Part model, mm, in its own coordinate system. A direction names the side the tool comes from. Round coordinates to 2 decimals unless told otherwise and drop trailing zeros. Write each loop counter-clockwise with the first axis right and the second up, starting at its lowest first coordinate (ties: lowest second). Pieces come first, ordered by that corner, then holes. Notation, with made-up numbers: (23, 71.5) -> (50, 71.5) arc R15 ccw to (50, 87.5) -> close; hole circle Ø10 at (-2.5, -38). An arc over 180 degrees is marked (long way). Use CSV: the item, a comma, the result in double quotes. Start each with the question number.
(1) Saw through at A-A (y = 231.5). Give the cut face in (x, z).
(2) Which spindle directions (+Z, -Z, +X, -X, +Y, -Y) get a long thin tool onto all of the face, cutting with end or side? Do faces 5 (the flat face through (51, 247, 0)), 6 (the flat face through (41.5, 321, 14)), 7 (the cylindrical face through (16.28, 46.49, 13.8)), 8 (the flat face through (61.5, 321, 14)). Say none if no direction does.
(3) Two-plate mould, pull along X, no slides. Class faces 1 (the flat face through (0, 24, 14)), 2 (the flat face through (51, 247, 28)), 3 (the flat face through (103, 24, 14)), 4 (the flat face through (51, 51, 14)): released by +X, released by -X, zero draft, split by the parting line, or undercut.
(4) Drop flat-ended pins along their axis: pin 1 (1.5 mm diameter, centred on x = 15.5, z = 17.5, fed in from -Y); pin 2 (14 mm diameter, centred on x = 59.5, z = 18.5, fed in from -Y); pin 3 (4 mm diameter, centred on x = 34.5, z = 3.5, fed in from +Y); pin 4 (5 mm diameter, centred on y = 8.5, z = 14, fed in from -X). Give the stop position or say it passes through.
(5) Probe line 1 (Z direction, x = 100, y = 8); line 2 (Y direction, x = 29, z = 20); line 3 (Y direction, x = 45.75, z = 14). List the from-to ranges inside material, lowest first. Write a range as [from, to].
```python
from build123d import *

# Parameters (mm, degrees)
BOSS_EXTRU_1_DEPTH      = 28
ESQUISSE2_R             = 3
ENL_V_MAT_EXTRU_1_DEPTH = 124.943535531
ESQUISSE3_W             = 20
ESQUISSE3_H             = 28
BOSS_EXTRU_2_DEPTH      = 524
CONG_1_SIZE             = 10
ESQUISSE4_R             = 4
ENL_V_MAT_EXTRU_2_DEPTH = 591.876679285


with BuildPart() as part:
    # Esquisse1 → Boss.-Extru.1 (new body)
    with BuildSketch(Plane.XY):
        with BuildLine():
            Line((27, 51), (51.5, 51))
            Line((51.5, 51), (51.5, 63))
            Line((51.5, 63), (15, 63))
            ThreePointArc((15, 63), (4.393398282, 58.606601718), (0, 48))
            Line((0, 48), (0, 0))
            Line((0, 0), (12, 0))
            Line((12, 0), (12, 36))
            ThreePointArc((12, 36), (16.393398282, 46.606601718), (27, 51))
        make_face()
        with BuildLine():
            Line((51.5, 63), (51.5, 51))
            Line((51.5, 51), (76, 51))
            ThreePointArc((76, 51), (86.606601718, 46.606601718), (91, 36))
            Line((91, 36), (91, 0))
            Line((91, 0), (103, 0))
            Line((103, 0), (103, 48))
            ThreePointArc((103, 48), (98.606601718, 58.606601718), (88, 63))
            Line((88, 63), (51.5, 63))
        make_face()
    extrude(amount=BOSS_EXTRU_1_DEPTH)

    # Esquisse2 → Enlèv. mat.-Extru.1 (cut, through all)
    with BuildSketch(Plane(origin=(103, 0, 0), x_dir=(0, 0, -1), z_dir=(1, 0, 0))):
        with Locations((-14, 8.5)):
            Circle(ESQUISSE2_R)
    extrude(amount=-ENL_V_MAT_EXTRU_1_DEPTH, mode=Mode.SUBTRACT)

    # Esquisse3 → Boss.-Extru.2 (add)
    with BuildSketch(Plane(origin=(0, 63, 0), x_dir=(1, 0, 0), z_dir=(0, 1, 0))):
        with Locations((51.5, -14)):
            Rectangle(ESQUISSE3_W, ESQUISSE3_H)
    extrude(amount=BOSS_EXTRU_2_DEPTH)

    # Congé1
    # a fillet whose section is not a circle: 10 mm, written as the material it takes off along each edge
    with BuildSketch(Plane(origin=(16.5, 587, 0), x_dir=(0, -1, 0), z_dir=(1, 0, 0)), Plane(origin=(86.5, 587, 28), x_dir=(0, -1, 0), z_dir=(-1, 0, 0))) as cong_1_piece_1:
        with BuildLine():
            Bezier((CONG_1_SIZE, 0), (0, 0), (0, -CONG_1_SIZE), weights=[1, 0.785674201, 1])
            Line((0, -CONG_1_SIZE), (0, 0))
            Line((0, 0), (CONG_1_SIZE, 0))
        make_face()
    extrude(amount=70, mode=Mode.SUBTRACT)

    # Esquisse4 → Enlèv. mat.-Extru.2 (cut, through all)
    with BuildSketch(Plane.ZY.offset(-41.5)):
        with Locations((14, 77)):
            Circle(ESQUISSE4_R)
    extrude(amount=-ENL_V_MAT_EXTRU_2_DEPTH, mode=Mode.SUBTRACT)


solid = part.part
```
Answers:
1,outline,"(41.5, 0) -> (61.5, 0) -> (61.5, 28) -> (41.5, 28) -> close"
2,face 5,"-Z, +X, -X, +Y, -Y"
2,face 6,"+Z, -Z, -X, +Y"
2,face 7,"+Z, -Z, -Y"
2,face 8,"+Z, -Z, +X, +Y"
3,face 1,"released by -X"
3,face 2,"zero draft"
3,face 3,"released by +X"
3,face 4,"undercut"
4,pin 1,"stops at y = 44.66"
4,pin 2,"stops at y = 51"
4,pin 3,"stops at y = 63"
4,pin 4,"passes through"
5,line 1,"z = [0, 11.04], [16.96, 28]"
5,line 2,"y = [51, 63]"
5,line 3,"y = [51, 73], [81, 587]"
